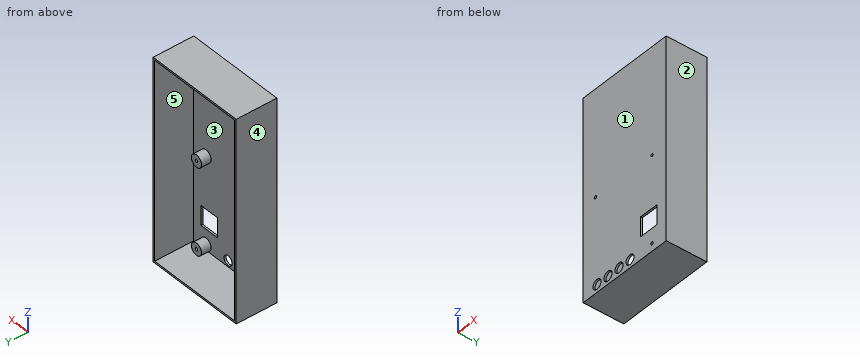
from build123d import *

# Parameters (mm, degrees)
SKETCH1_W            = 64.516
SKETCH1_H            = 133.223
SKETCH1_R            = 3.25
SKETCH1_R_2          = 0.9652
SKETCH1_W_2          = 13.208
SKETCH1_H_2          = 13.208
FRONT_FACE_DEPTH     = 1.27
SKETCH2_R            = 4.1275
SKETCH2_R_2          = 0.9652
SKETCH2_R_3          = 4.064
SCREW_POST_PCB_DEPTH = 6.5
SKETCH5_W            = 1.27
SKETCH5_H            = 27.432
SIDE_WALLS_DEPTH     = 133.223
SKETCH6_W            = 1.27
SKETCH6_H            = 27.432
BOTTOM_WALL_DEPTH    = 67.056
SKETCH8_W            = 67.056
SKETCH8_H            = 27.432
TOP_WALL_DEPTH       = 1.27


with BuildPart() as part:
    # Sketch1 → front_face (new body)
    with BuildSketch(Plane(origin=(0, 0, 0), x_dir=(1, 0, 0), z_dir=(0, 1, 0))):
        with Locations((51.562, 6.096)):
            Rectangle(SKETCH1_W, SKETCH1_H)
        with Locations(Location((29.21, 68.58, 0), (0, 0, 270))):
            Circle(SKETCH1_R, mode=Mode.SUBTRACT)
        with Locations(Location((38.1, 68.58, 0), (0, 0, 270))):
            Circle(SKETCH1_R, mode=Mode.SUBTRACT)
        with Locations(Location((46.99, 68.58, 0), (0, 0, 270))):
            Circle(SKETCH1_R, mode=Mode.SUBTRACT)
        with Locations(Location((55.88, 68.58, 0), (0, 0, 270))):
            Circle(SKETCH1_R, mode=Mode.SUBTRACT)
        with Locations(Location((73.66, 68.58, 0), (0, 0, 270))):
            Circle(SKETCH1_R_2, mode=Mode.SUBTRACT)
        with Locations(Location((73.66, 10.16, 0), (0, 0, 270))):
            Circle(SKETCH1_R_2, mode=Mode.SUBTRACT)
        with Locations(Location((27.94, 10.16, 0), (0, 0, 270))):
            Circle(SKETCH1_R_2, mode=Mode.SUBTRACT)
        with Locations((71.12, 52.07)):
            Rectangle(SKETCH1_W_2, SKETCH1_H_2, mode=Mode.SUBTRACT)
    extrude(amount=FRONT_FACE_DEPTH)

    # Sketch2 → screw_post_PCB (add)
    # profile 1 of 3: a face of its own
    with BuildSketch(Plane(origin=(0, 1.27, 0), x_dir=(1, 0, 0), z_dir=(0, 1, 0))):
        with Locations(Location((27.94, 10.16, 0), (0, 0, 90))):
            Circle(SKETCH2_R)
        with Locations(Location((27.94, 10.16, 0), (0, 0, 270))):
            Circle(SKETCH2_R_2, mode=Mode.SUBTRACT)
    # profile 2 of 3: a face of its own
    with BuildSketch(Plane(origin=(0, 1.27, 0), x_dir=(1, 0, 0), z_dir=(0, 1, 0))):
        with Locations(Location((73.66, 10.16, 0), (0, 0, 90))):
            Circle(SKETCH2_R)
        with Locations(Location((73.66, 10.16, 0), (0, 0, 270))):
            Circle(SKETCH2_R_2, mode=Mode.SUBTRACT)
    # profile 3 of 3: a face of its own
    with BuildSketch(Plane(origin=(0, 1.27, 0), x_dir=(1, 0, 0), z_dir=(0, 1, 0))):
        with Locations(Location((73.66, 68.58, 0), (0, 0, 90))):
            Circle(SKETCH2_R_3)
        with Locations(Location((73.66, 68.58, 0), (0, 0, 270))):
            Circle(SKETCH2_R_2, mode=Mode.SUBTRACT)
    extrude(amount=SCREW_POST_PCB_DEPTH)

    # Sketch5 → side_walls (add)
    with BuildSketch(Plane(origin=(0, 0, -72.7075), x_dir=(-1, 0, 0), z_dir=(0, 0, -1))):
        with Locations((-84.455, 13.716)):
            Rectangle(SKETCH5_W, SKETCH5_H)
        with Locations((-18.669, 13.716)):
            Rectangle(SKETCH5_W, SKETCH5_H)
    extrude(amount=-SIDE_WALLS_DEPTH)

    # Sketch6 → bottom_wall (add)
    with BuildSketch(Plane(origin=(85.09, 0, 0), x_dir=(0, 0, -1), z_dir=(1, 0, 0))):
        with Locations((-61.1505, 13.716)):
            Rectangle(SKETCH6_W, SKETCH6_H)
    extrude(amount=-BOTTOM_WALL_DEPTH)

    # Sketch8 → top_wall (add)
    with BuildSketch(Plane(origin=(0, 0, -72.7075), x_dir=(-1, 0, 0), z_dir=(0, 0, -1))):
        with Locations((-51.562, 13.716)):
            Rectangle(SKETCH8_W, SKETCH8_H)
    extrude(amount=TOP_WALL_DEPTH)


solid = part.part
Geometry: final body of the model. Coordinates: model frame, mm. Face numbers are marked on the shaded views. A direction names the side the tool comes from. Coordinates: 2 decimals unless noted, no trailing zeros. Loops run counter-clockwise (first coordinate to the right, second up) from the corner with the lowest first, then second, coordinate; pieces in that order, holes last. Notation, with made-up numbers: (89, 42.25) - (132, 42.25) arc R23 ccw to (132, 60.25) - close; hole circle Ø5 at (39, 10.25). An arc over 180 degrees is marked (long way). One line per question, with ' | ' between items. Start each with the question number.
(1) Cut plane D-D on z = 43.5. Output: boundary loops of the cut face in (x, y).
(2) Cut plane C-C on y = 21.5. Output: boundary loops of the cut face in (x, z), and give its area (3 significant figures).
(3) Draft query along X for the marked faces 1, 2 and 3. Return one class per face: +X half, -X half, draft (parallel to the pull), parting line (faces both ways), or undercut.
(4) Ray query, L1, parallel to X at y = 0.9, z = -68.58; L2, parallel to X at y = 2, z = -10.16; L3, parallel to Z at x = 64.5, y = 13.5. Return the intervals inside material, ascending. Write a range as from..to.
(5) Cut plane B-B on x = 38.1. Output: boundary loops of the cut face in (y, z), and give its area (3 significant figures).
(6) Reachability of the marked faces 4 and 5 from +Z, -Z, +X, -X, +Y, -Y: full face, straight path, thin tool, end or side. Return the list, or none.
(7) Cut plane A-A on y = 5.75. Output: boundary loops of the cut face in (x, z) (1 decimal).
(8) First-contact query: pin 1 (4 mm diameter, centred on x = 75.5, z = -68.5, fed in from +Y); pin 2 (5 mm diameter, centred on x = 38.1, z = -68.58, fed in from -Y); pin 3 (4 mm diameter, centred on x = 26.5, z = -31, fed in from +Y). Flat tips, straight axial feed; report the tip coordinate or a pass-through.
Here are the results:
1) outline: (18.03, 0) - (85.09, 0) - (85.09, 27.43) - (83.82, 27.43) - (83.82, 1.27) - (19.3, 1.27) - (19.3, 27.43) - (18.03, 27.43) - close
2) outline: (18.03, -73.98) - (85.09, -73.98) - (85.09, 61.79) - (18.03, 61.79) - close; hole (19.3, -72.71) - (83.82, -72.71) - (83.82, 60.52) - (19.3, 60.52) - close | area: 509 mm²
3) face 1: draft | face 2: +X half | face 3: undercut
4) L1: 18.03..25.96, 32.46..34.85, 41.35..43.74, 50.24..52.63, 59.13..72.69, 74.63..85.09 | L2: 18.03..19.3, 23.81..26.97, 28.91..32.07, 69.53..72.69, 74.63..77.79, 83.82..85.09 | L3: -73.98..-72.71, 60.52..61.79
5) outline: (0, -73.98) - (27.43, -73.98) - (27.43, -72.71) - (1.27, -72.71) - (1.27, -71.83) - (0, -71.83) - close; (0, -65.33) - (1.27, -65.33) - (1.27, 60.52) - (27.43, 60.52) - (27.43, 61.79) - (0, 61.79) - close | area: 231 mm²
6) face 4: +Z, -Z, -X, +Y, -Y | face 5: +Y
7) outline: (18, -74) - (85.1, -74) - (85.1, 61.8) - (18, 61.8) - close; circle Ø8.3 at (27.9, -10.2); circle Ø8.3 at (73.7, -10.2); circle Ø8.1 at (73.7, -68.6); hole (19.3, -72.7) - (83.8, -72.7) - (83.8, 60.5) - (19.3, 60.5) - close; hole circle Ø1.9 at (27.9, -10.2); hole circle Ø1.9 at (73.7, -68.6); hole circle Ø1.9 at (73.7, -10.2)
8) pin 1: y = 7.77 | pin 2: through | pin 3: y = 1.27
